Part model, mm, in its own coordinate system. Give positions to 0.01 mm unless a question says otherwise; leave off trailing zeros. Order: outer loops, then holes, each group sorted by start corner. A loop starts at its lowest first (then second) coordinate and runs counter-clockwise, first axis right, second up. Notation, with made-up numbers: (71.25, 87.5) - (79.25, 87.5) arc R7 cw to (79.25, 96.5) - close; hole circle Ø10 at (-10.5, 62.5). An arc over 180 degrees is marked (long way). One line per item, written item: value.
```python
from build123d import *

# Parameters (mm, degrees)
SKETCH1_R           = 3.4925
BOSS_EXTRUDE1_DEPTH = 44.45


with BuildPart() as part:
    # Sketch1 → Boss-Extrude1 (new body, symmetric)
    with BuildSketch(Plane(origin=(0, 0, 0), x_dir=(0, 0, -1), z_dir=(1, 0, 0))):
        with BuildLine():
            Line((-25.4, -6.35), (25.4, -6.35))
            ThreePointArc((25.4, -6.35), (31.75, 0), (25.4, 6.35))
            Line((25.4, 6.35), (-25.4, 6.35))
            ThreePointArc((-25.4, 6.35), (-31.75, 0), (-25.4, -6.35))
        make_face()
        with Locations((-25.4, 0)):
            Circle(SKETCH1_R, mode=Mode.SUBTRACT)
        with Locations((25.4, 0)):
            Circle(SKETCH1_R, mode=Mode.SUBTRACT)
        Circle(SKETCH1_R, mode=Mode.SUBTRACT)
    extrude(amount=BOSS_EXTRUDE1_DEPTH, both=True)


solid = part.part
```
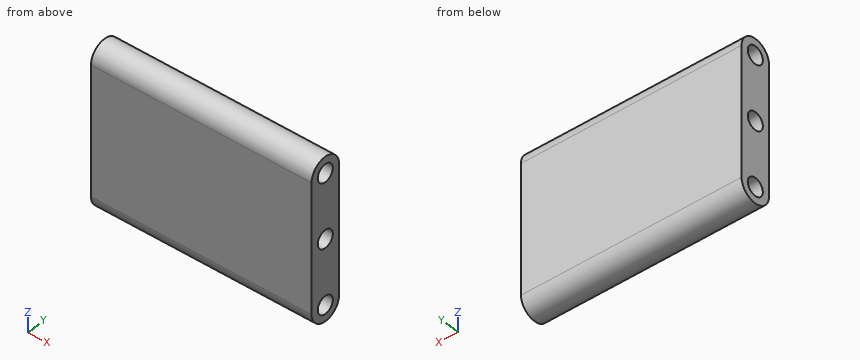
1) Cut at A-A, the plane x = -4.5. Give the number of separate pieces and of enclosed holes in the cut face, then the cut area to 3 significant figures.
Outcome:
separate pieces: 1
enclosed holes: 3
area: 657 mm^2
2) Cut at D-D, the plane y = 4.5. Give the cut face in (x, z), then the cut area to 3 significant figures.
Outcome:
outline: (-44.45, -29.88) - (44.45, -29.88) - (44.45, 29.88) - (-44.45, 29.88) - close
area: 5,310 mm^2
3) Drill centre lines: line 1 along Y through (x, z) = (12.5, 25.4); line 2 along Z through (x, y) = (22, -1.5); line 3 along Z through (x, y) = (21, 1.75). Where is each one in solid material? Low to high. Write a range as from..to.
Outcome:
line 1: y = -6.35..-3.49, 3.49..6.35
line 2: z = -31.57..-28.55, -22.25..-3.15, 3.15..22.25, 28.55..31.57
line 3: z = -31.5..-28.42, -22.38..-3.02, 3.02..22.38, 28.42..31.5
4) Cut at C-C, the plane y = -2.5. Give the cut face in (x, z).
Outcome:
outline: (-44.45, -31.24) - (44.45, -31.24) - (44.45, -27.84) - (-44.45, -27.84) - close; (-44.45, -22.96) - (44.45, -22.96) - (44.45, -2.44) - (-44.45, -2.44) - close; (-44.45, 2.44) - (44.45, 2.44) - (44.45, 22.96) - (-44.45, 22.96) - close; (-44.45, 27.84) - (44.45, 27.84) - (44.45, 31.24) - (-44.45, 31.24) - close
5) Pin check, flat tips, straight feed: pin 1 (3 mm diameter, centred on x = 1.5, y = 5, fed in from +Z); pin 2 (1 mm diameter, centred on x = -2, y = 3.5, fed in from -Z). Stop position of each tip, or through.
Outcome:
pin 1: stops at z = 30.7
pin 2: stops at z = -31
6) Cut at B-B, the plane z = 0. Give the cut face in (x, y), then the cut area to 3 significant figures.
Outcome:
outline: (-44.45, -6.35) - (44.45, -6.35) - (44.45, -3.49) - (-44.45, -3.49) - close; (-44.45, 3.49) - (44.45, 3.49) - (44.45, 6.35) - (-44.45, 6.35) - close
area: 508 mm^2
